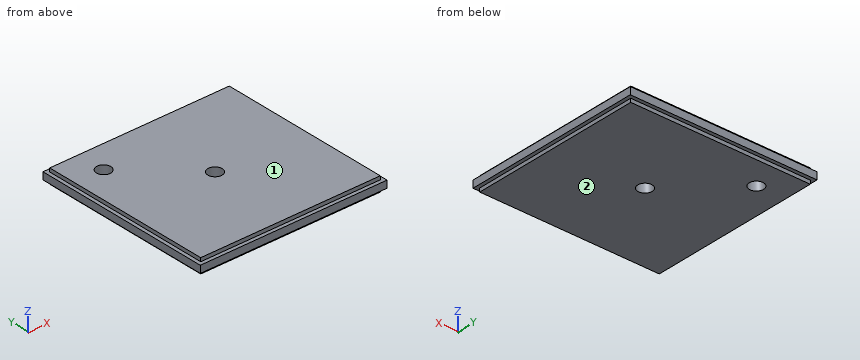
from build123d import *

# Parameters (mm, degrees)
F0_W      = 317.5
F0_H      = 304.8
F1_DEPTH  = 25.4
F2_W      = 317.5
F2_H      = 12.7
F3_DEPTH  = 6.35
F4_W      = 317.5
F4_H      = 12.7
F5_DEPTH  = 6.35
F8_DEPTH  = 6.35
F9_DEPTH  = 6.35
F10_R     = 12.7
F11_DEPTH = 25.4
F12_R     = 12.7
F13_DEPTH = 25.4


with BuildPart() as f1:
    # F0 (on Top) → F1 (new body)
    with BuildSketch(Plane.XY):
        Rectangle(F0_W, F0_H)
    extrude(amount=F1_DEPTH)

    # F2 (on face) → F3 (join)
    with BuildSketch(Plane.XZ.offset(152.4)):
        with Locations((0, 12.7)):
            Rectangle(F2_W, F2_H)
    extrude(amount=F3_DEPTH)

    # F4 (on face) → F5 (join)
    with BuildSketch(Plane(origin=(0, 152.4, 0), x_dir=(-1, 0, 0), z_dir=(0, 1, 0))):
        with Locations((0, 12.7)):
            Rectangle(F4_W, F4_H)
    extrude(amount=F5_DEPTH)

    # F7 (on face) → F8 (join)
    with BuildSketch(Plane(origin=(-158.75, 0, 0), x_dir=(0, -1, 0), z_dir=(-1, 0, 0))):
        Polygon((-152.4, 19.05), (-158.75, 19.05), (-158.75, 6.35), (-152.4, 6.35), (152.4, 6.35), (158.75, 6.35), (158.75, 19.05), (152.4, 19.05), align=None)
    extrude(amount=F8_DEPTH)

    # F6 (on face) → F9 (join)
    with BuildSketch(Plane.YZ.offset(158.75)):
        Polygon((-152.4, 19.05), (-158.75, 19.05), (-158.75, 6.35), (-152.4, 6.35), (152.4, 6.35), (158.75, 6.35), (158.75, 19.05), (152.4, 19.05), align=None)
    extrude(amount=F9_DEPTH)

    # F10 (on face) → F11 (cut)
    with BuildSketch(Plane.XY.offset(25.4)):
        with Locations((-107.95, 101.6)):
            Circle(F10_R)
    extrude(amount=-F11_DEPTH, mode=Mode.SUBTRACT)

    # F12 (on face) → F13 (cut)
    with BuildSketch(Plane.XY.offset(25.4)):
        Circle(F12_R)
    extrude(amount=-F13_DEPTH, mode=Mode.SUBTRACT)


solid = f1.part
For this review, take the finished solid that the model builds, in its own axes (mm). Face numbers are marked on the shaded views. Give positions to 0.01 mm unless a question says otherwise; leave off trailing zeros. Loops run counter-clockwise (first coordinate to the right, second up) from the corner with the lowest first, then second, coordinate; pieces in that order, holes last.
Item 1: Take a section at A-A, the plane y = 101.6. State the section outline as (x, z) points, and give its area (3 significant figures).
Item 2: Take a section at C-C, the plane x = -56.5. State the section outline as (y, z) points, and give its area (3 significant figures).
Item 3: Insertion check: pin 1 (12 mm diameter, centred on x = -73, z = 3, fed in from +Y); pin 2 (1.9 mm diameter, centred on x = -44, z = 2, fed in from +Y); pin 3 (5 mm diameter, centred on x = -65.5, z = 3, fed in from -Y); pin 4 (3 mm diameter, centred on y = 80, z = 22, fed in from -X). Each pin has a flat end and moves straight along its axis. Give the tip position at first contact, or say it passes through.
Item 4: Draft analysis for pull direction Z (two halves, no side actions). For the marked faces 1 and 2, state which applies: +Z half, -Z half, draft (parallel to the pull), parting line (faces both ways), or undercut.
Item 5: For line 1 along Y through (x, z) = (-107.95, 11.5); line 2 along Y through (x, z) = (-107.95, 5.75); line 3 along Y through (x, z) = (98.5, 22.75), list the stretches that pass through material, from the lowest coordinate up.
Item 6: Take a section at D-D, the plane y = -45.5. State the section outline as (x, z) points, and give its area (3 significant figures).
Item 7: Take a section at B-B, the plane x = 0. State the section outline as (y, z) points.
Calculated:
1. outline: (-165.1, 6.35) - (-158.75, 6.35) - (-158.75, 0) - (-120.65, 0) - (-120.65, 25.4) - (-158.75, 25.4) - (-158.75, 19.05) - (-165.1, 19.05) - close; (-95.25, 0) - (158.75, 0) - (158.75, 6.35) - (165.1, 6.35) - (165.1, 19.05) - (158.75, 19.05) - (158.75, 25.4) - (-95.25, 25.4) - close
1. area: 7,580 mm2
2. outline: (-158.75, 6.35) - (-152.4, 6.35) - (-152.4, 0) - (152.4, 0) - (152.4, 6.35) - (158.75, 6.35) - (158.75, 19.05) - (152.4, 19.05) - (152.4, 25.4) - (-152.4, 25.4) - (-152.4, 19.05) - (-158.75, 19.05) - close
2. area: 7,900 mm2
3. pin 1: stops at y = 158.75
3. pin 2: stops at y = 152.4
3. pin 3: stops at y = -152.4
3. pin 4: stops at x = -158.75
4. face 1: +Z half
4. face 2: -Z half
5. line 1: y = -158.75 to 88.9, 114.3 to 158.75
5. line 2: y = -152.4 to 88.9, 114.3 to 152.4
5. line 3: y = -152.4 to 152.4
6. outline: (-165.1, 6.35) - (-158.75, 6.35) - (-158.75, 0) - (158.75, 0) - (158.75, 6.35) - (165.1, 6.35) - (165.1, 19.05) - (158.75, 19.05) - (158.75, 25.4) - (-158.75, 25.4) - (-158.75, 19.05) - (-165.1, 19.05) - close
6. area: 8,230 mm2
7. outline: (-158.75, 6.35) - (-152.4, 6.35) - (-152.4, 0) - (-12.7, 0) - (-12.7, 25.4) - (-152.4, 25.4) - (-152.4, 19.05) - (-158.75, 19.05) - close; (12.7, 0) - (152.4, 0) - (152.4, 6.35) - (158.75, 6.35) - (158.75, 19.05) - (152.4, 19.05) - (152.4, 25.4) - (12.7, 25.4) - close
